Can you work these out from the model? Positions are in its coordinate system, mm. Give positions to 0.01 mm unless a question says otherwise; leave off trailing zeros. Loops run counter-clockwise (first coordinate to the right, second up) from the corner with the lowest first, then second, coordinate; pieces in that order, holes last. Notation, with made-up numbers: (11.25, -27) - (44.25, -27) arc R12 ccw to (44.25, -10) - close; hole circle Ø4 at (22, 82.5). An arc over 180 degrees is marked (long way). Write item = value, one per line.
from build123d import *

# Parameters (mm, degrees)
SKETCH1_W            = 52
SKETCH1_H            = 40
SKETCH1_R            = 2.75
BOSS_EXTRUDE10_DEPTH = 5
SKETCH1_21_R         = 2.75
BOSS_EXTRUDE13_DEPTH = 5
SKETCH1_22_R         = 2.12
CUT_EXTRUDE4_DEPTH   = 7
CHAMFER1_SIZE        = 1
SKETCH1_23_R         = 2.75
BOSS_EXTRUDE14_DEPTH = 5
SKETCH1_24_R         = 2.12
CUT_EXTRUDE6_DEPTH   = 5
SKETCH1_25_R         = 2.75
BOSS_EXTRUDE15_DEPTH = 5
SKETCH1_26_R         = 2.12
CUT_EXTRUDE7_DEPTH   = 18
SKETCH1_29_R         = 2.75
BOSS_EXTRUDE17_DEPTH = 5
SKETCH1_30_R         = 2.12
CUT_EXTRUDE9_DEPTH   = 14
CHAMFER3_SIZE        = 1
CHAMFER4_SIZE        = 1
CHAMFER5_SIZE        = 1


with BuildPart() as part:
    # Sketch1 → Boss-Extrude10 (new body)
    with BuildSketch(Plane(origin=(0, 0, 0), x_dir=(1, 0, 0), z_dir=(0, 1, 0))):
        Rectangle(SKETCH1_W, SKETCH1_H)
        with Locations(Location((-20, 4, 0), (0, 0, 270))):
            Circle(SKETCH1_R, mode=Mode.SUBTRACT)
        with Locations(Location((20, 4, 0), (0, 0, 270))):
            Circle(SKETCH1_R, mode=Mode.SUBTRACT)
        with Locations(Location((-20, -12, 0), (0, 0, 270))):
            Circle(SKETCH1_R, mode=Mode.SUBTRACT)
        with Locations(Location((20, -12, 0), (0, 0, 270))):
            Circle(SKETCH1_R, mode=Mode.SUBTRACT)
    extrude(amount=BOSS_EXTRUDE10_DEPTH)

    # Sketch1_21 → Boss-Extrude13 (add)
    with BuildSketch(Plane(origin=(0, 0, 0), x_dir=(1, 0, 0), z_dir=(0, 1, 0))):
        with Locations((20, 4)):
            Circle(SKETCH1_21_R)
    extrude(amount=BOSS_EXTRUDE13_DEPTH)

    # Sketch1_22 → Cut-Extrude4 (cut)
    with BuildSketch(Plane(origin=(0, 0, 0), x_dir=(1, 0, 0), z_dir=(0, 1, 0))):
        with Locations(Location((20, 4, 0), (0, 0, 90))):
            Circle(SKETCH1_22_R)
    extrude(amount=CUT_EXTRUDE4_DEPTH, mode=Mode.SUBTRACT)

    # Chamfer1
    chamfer1_edges = [part.edges().sort_by_distance(p)[0] for p in [
        (20, 5, -1.88),
    ]]
    chamfer(chamfer1_edges, length=CHAMFER1_SIZE)

    # Sketch1_23 → Boss-Extrude14 (add)
    with BuildSketch(Plane(origin=(0, 0, 0), x_dir=(1, 0, 0), z_dir=(0, 1, 0))):
        with Locations((20, -12)):
            Circle(SKETCH1_23_R)
    extrude(amount=BOSS_EXTRUDE14_DEPTH)

    # Sketch1_24 → Cut-Extrude6 (cut)
    with BuildSketch(Plane(origin=(0, 0, 0), x_dir=(1, 0, 0), z_dir=(0, 1, 0))):
        with Locations(Location((20, -12, 0), (0, 0, 90))):
            Circle(SKETCH1_24_R)
    extrude(amount=CUT_EXTRUDE6_DEPTH, mode=Mode.SUBTRACT)

    # Sketch1_25 → Boss-Extrude15 (add)
    with BuildSketch(Plane(origin=(0, 0, 0), x_dir=(1, 0, 0), z_dir=(0, 1, 0))):
        with Locations((-20, -12)):
            Circle(SKETCH1_25_R)
    extrude(amount=BOSS_EXTRUDE15_DEPTH)

    # Sketch1_26 → Cut-Extrude7 (cut)
    with BuildSketch(Plane(origin=(0, 0, 0), x_dir=(1, 0, 0), z_dir=(0, 1, 0))):
        with Locations(Location((-20, -12, 0), (0, 0, 270))):
            Circle(SKETCH1_26_R)
    extrude(amount=CUT_EXTRUDE7_DEPTH, mode=Mode.SUBTRACT)

    # Sketch1_29 → Boss-Extrude17 (add)
    with BuildSketch(Plane(origin=(0, 0, 0), x_dir=(1, 0, 0), z_dir=(0, 1, 0))):
        with Locations((-20, 4)):
            Circle(SKETCH1_29_R)
    extrude(amount=BOSS_EXTRUDE17_DEPTH)

    # Sketch1_30 → Cut-Extrude9 (cut)
    with BuildSketch(Plane(origin=(0, 0, 0), x_dir=(1, 0, 0), z_dir=(0, 1, 0))):
        with Locations(Location((-20, 4, 0), (0, 0, 270))):
            Circle(SKETCH1_30_R)
    extrude(amount=CUT_EXTRUDE9_DEPTH, mode=Mode.SUBTRACT)

    # Chamfer3
    chamfer3_edges = [part.edges().sort_by_distance(p)[0] for p in [
        (-20, 5, -6.12),
    ]]
    chamfer(chamfer3_edges, length=CHAMFER3_SIZE)

    # Chamfer4
    chamfer4_edges = [part.edges().sort_by_distance(p)[0] for p in [
        (-20, 5, 9.88),
    ]]
    chamfer(chamfer4_edges, length=CHAMFER4_SIZE)

    # Chamfer5
    chamfer5_edges = [part.edges().sort_by_distance(p)[0] for p in [
        (20, 5, 14.12),
    ]]
    chamfer(chamfer5_edges, length=CHAMFER5_SIZE)


solid = part.part
Q1. I need wall thicknesses on L1, parallel to Z at x = 20, y = 1.05; L2, parallel to X at y = 1.6, z = 12; L3, parallel to X at y = 3.7, z = -3. Which ranges of each line are inside material? Lowest first, please.
Output:
L1 = -20 to -6.12, -1.88 to 9.88, 14.12 to 20
L2 = -26 to -22.12, -17.88 to 17.88, 22.12 to 26
L3 = -26 to -21.87, -18.13 to 18.13, 21.87 to 26
Q2. For pin 1 (3.5 mm diameter, centred on x = -20, z = 12, fed in from -Y); pin 2 (2 mm diameter, centred on x = 16.5, z = -15.5, fed in from -Y), each with a flat end and sliding along its axis, tell me the tip position at first contact or that it passes through.
Output:
pin_1 = through
pin_2 = 0
Q3. Imagine slicing it at B-B, the plane x = 20. Write out the boundary of the cut face in (y, z).
Output:
outline = (0, -20) - (5, -20) - (5, -7.12) - (4, -6.12) - (0, -6.12) - close; (0, -1.88) - (4, -1.88) - (5, -0.88) - (5, 8.88) - (4, 9.88) - (0, 9.88) - close; (0, 14.12) - (4, 14.12) - (5, 15.12) - (5, 20) - (0, 20) - close
Q4. Imagine slicing it at C-C, the plane y = 1.5. Write out the boundary of the cut face in (x, z).
Output:
outline = (-26, -20) - (26, -20) - (26, 20) - (-26, 20) - close; hole circle Ø4.24 at (-20, -4); hole circle Ø4.24 at (-20, 12); hole circle Ø4.24 at (20, -4); hole circle Ø4.24 at (20, 12)
Q5. Imagine slicing it at A-A, the plane z = 12. Write out the boundary of the cut face in (x, y).
Output:
outline = (-26, 0) - (-22.12, 0) - (-22.12, 4) - (-23.12, 5) - (-26, 5) - close; (-17.88, 0) - (17.88, 0) - (17.88, 4) - (16.88, 5) - (-16.88, 5) - (-17.88, 4) - close; (22.12, 0) - (26, 0) - (26, 5) - (23.12, 5) - (22.12, 4) - close
Q6. We'd pull the mould along Z, two halves only. Please class faces 1 (the flat face through (0, 2, -20)), 2 (the cylindrical face through (-20.81, 1.97, 13.96)), 3 (the flat face through (0, 5, 0)): released by +Z, released by -Z, zero draft, split by the parting line, or undercut.
Output:
face_1 = released by -Z
face_2 = undercut
face_3 = zero draft
